Build history of the part. All positions in model axes, mm. A direction names the side the tool comes from. Round coordinates to 2 decimals unless told otherwise and drop trailing zeros. Loops run counter-clockwise (first coordinate to the right, second up) from the corner with the lowest first, then second, coordinate; pieces in that order, holes last. Notation, with made-up numbers: (59.5, 48) - (112.5, 48) arc R11 ccw to (112.5, 66) - close; hole circle Ø6 at (66.5, 42.25). An arc over 180 degrees is marked (long way). Put each result on its own line as item: value. Start each with the question number.
from build123d import *

# Parameters (mm, degrees)
SKETCH2_R                            = 3.35
F_40_SERIES_TS40_80LM_650037_1_DEPTH = 175


with BuildPart() as part:
    # Sketch2 → 40 series TS40-80LM-650037(1) (new body)
    with BuildSketch(Plane(origin=(0, 0, 0), x_dir=(-1, 0, 0), z_dir=(0, 1, 0))):
        with BuildLine():
            Line((0, -27.681), (-5.525738531, -27.681))
            Line((-5.525738531, -27.681), (-11.176, -33.331261469))
            Line((-11.176, -33.331261469), (-11.176, -36.6218))
            Line((-11.176, -36.6218), (-7.6835, -36.6218))
            Line((-7.6835, -36.6218), (-7.6835, -35.2248))
            Line((-7.6835, -35.2248), (-4.0488, -35.2248))
            Line((-4.0488, -35.2248), (-4.0488, -40))
            Line((-4.0488, -40), (-17, -40))
            ThreePointArc((-17, -40), (-19.121320344, -39.121320344), (-20, -37))
            Line((-20, -37), (-20, -24.0488))
            Line((-20, -24.0488), (-15.2248, -24.0488))
            Line((-15.2248, -24.0488), (-15.2248, -27.6835))
            Line((-15.2248, -27.6835), (-16.6218, -27.6835))
            Line((-16.6218, -27.6835), (-16.6218, -31.176))
            Line((-16.6218, -31.176), (-13.331261469, -31.176))
            Line((-13.331261469, -31.176), (-7.681, -25.525738531))
            Line((-7.681, -25.525738531), (-7.681, -20))
            Line((-7.681, -20), (-7.681, -14.474261469))
            Line((-7.681, -14.474261469), (-13.331261469, -8.824))
            Line((-13.331261469, -8.824), (-16.6218, -8.824))
            Line((-16.6218, -8.824), (-16.6218, -12.3165))
            Line((-16.6218, -12.3165), (-15.2248, -12.3165))
            Line((-15.2248, -12.3165), (-15.2248, -15.9512))
            Line((-15.2248, -15.9512), (-20, -15.9512))
            Line((-20, -15.9512), (-20, 15.9512))
            Line((-20, 15.9512), (-15.2248, 15.9512))
            Line((-15.2248, 15.9512), (-15.2248, 12.3165))
            Line((-15.2248, 12.3165), (-16.6218, 12.3165))
            Line((-16.6218, 12.3165), (-16.6218, 8.824))
            Line((-16.6218, 8.824), (-13.331261469, 8.824))
            Line((-13.331261469, 8.824), (-7.681, 14.474261469))
            Line((-7.681, 14.474261469), (-7.681, 25.525738531))
            Line((-7.681, 25.525738531), (-13.331261469, 31.176))
            Line((-13.331261469, 31.176), (-16.6218, 31.176))
            Line((-16.6218, 31.176), (-16.6218, 27.6835))
            Line((-16.6218, 27.6835), (-15.2248, 27.6835))
            Line((-15.2248, 27.6835), (-15.2248, 24.0488))
            Line((-15.2248, 24.0488), (-20, 24.0488))
            Line((-20, 24.0488), (-20, 37))
            ThreePointArc((-20, 37), (-19.121320344, 39.121320344), (-17, 40))
            Line((-17, 40), (-4.0488, 40))
            Line((-4.0488, 40), (-4.0488, 35.2248))
            Line((-4.0488, 35.2248), (-7.6835, 35.2248))
            Line((-7.6835, 35.2248), (-7.6835, 36.6218))
            Line((-7.6835, 36.6218), (-11.176, 36.6218))
            Line((-11.176, 36.6218), (-11.176, 33.331261469))
            Line((-11.176, 33.331261469), (-5.525738531, 27.681))
            Line((-5.525738531, 27.681), (0, 27.681))
            Line((0, 27.681), (5.525738531, 27.681))
            Line((5.525738531, 27.681), (11.176, 33.331261469))
            Line((11.176, 33.331261469), (11.176, 36.6218))
            Line((11.176, 36.6218), (7.6835, 36.6218))
            Line((7.6835, 36.6218), (7.6835, 35.2248))
            Line((7.6835, 35.2248), (4.0488, 35.2248))
            Line((4.0488, 35.2248), (4.0488, 40))
            Line((4.0488, 40), (17, 40))
            ThreePointArc((17, 40), (19.121320344, 39.121320344), (20, 37))
            Line((20, 37), (20, 24.0488))
            Line((20, 24.0488), (15.2248, 24.0488))
            Line((15.2248, 24.0488), (15.2248, 27.6835))
            Line((15.2248, 27.6835), (16.6218, 27.6835))
            Line((16.6218, 27.6835), (16.6218, 31.176))
            Line((16.6218, 31.176), (13.331261469, 31.176))
            Line((13.331261469, 31.176), (7.681, 25.525738531))
            Line((7.681, 25.525738531), (7.681, 20))
            Line((7.681, 20), (7.681, 14.474261469))
            Line((7.681, 14.474261469), (13.331261469, 8.824))
            Line((13.331261469, 8.824), (16.6218, 8.824))
            Line((16.6218, 8.824), (16.6218, 12.3165))
            Line((16.6218, 12.3165), (15.2248, 12.3165))
            Line((15.2248, 12.3165), (15.2248, 15.9512))
            Line((15.2248, 15.9512), (20, 15.9512))
            Line((20, 15.9512), (20, -15.9512))
            Line((20, -15.9512), (15.2248, -15.9512))
            Line((15.2248, -15.9512), (15.2248, -12.3165))
            Line((15.2248, -12.3165), (16.6218, -12.3165))
            Line((16.6218, -12.3165), (16.6218, -8.824))
            Line((16.6218, -8.824), (13.331261469, -8.824))
            Line((13.331261469, -8.824), (7.681, -14.474261469))
            Line((7.681, -14.474261469), (7.681, -20))
            Line((7.681, -20), (7.681, -25.525738531))
            Line((7.681, -25.525738531), (13.331261469, -31.176))
            Line((13.331261469, -31.176), (16.6218, -31.176))
            Line((16.6218, -31.176), (16.6218, -27.6835))
            Line((16.6218, -27.6835), (15.2248, -27.6835))
            Line((15.2248, -27.6835), (15.2248, -24.0488))
            Line((15.2248, -24.0488), (20, -24.0488))
            Line((20, -24.0488), (20, -37))
            ThreePointArc((20, -37), (19.121320344, -39.121320344), (17, -40))
            Line((17, -40), (4.0488, -40))
            Line((4.0488, -40), (4.0488, -35.2248))
            Line((4.0488, -35.2248), (7.6835, -35.2248))
            Line((7.6835, -35.2248), (7.6835, -36.6218))
            Line((7.6835, -36.6218), (11.176, -36.6218))
            Line((11.176, -36.6218), (11.176, -33.331261469))
            Line((11.176, -33.331261469), (5.525738531, -27.681))
            Line((5.525738531, -27.681), (0, -27.681))
        make_face()
        with Locations((0, -20)):
            Circle(SKETCH2_R, mode=Mode.SUBTRACT)
        with Locations((0, 20)):
            Circle(SKETCH2_R, mode=Mode.SUBTRACT)
        Polygon((-5.525738531, 12.319), (-17.844738531, 0), (-5.525738531, -12.319), (0, -12.319), (5.525738531, -12.319), (17.844738531, 0), (5.525738531, 12.319), (0, 12.319), align=None, mode=Mode.SUBTRACT)
        with BuildLine():
            Line((12.8372, 38.222), (12.8372, 32.8372))
            Line((12.8372, 32.8372), (18.222, 32.8372))
            Line((18.222, 32.8372), (18.222, 35.428))
            ThreePointArc((18.222, 35.428), (17.403656347, 37.403656347), (15.428, 38.222))
            Line((15.428, 38.222), (12.8372, 38.222))
        make_face(mode=Mode.SUBTRACT)
        with BuildLine():
            Line((12.8372, -32.8372), (18.222, -32.8372))
            Line((18.222, -32.8372), (18.222, -35.428))
            ThreePointArc((18.222, -35.428), (17.403656347, -37.403656347), (15.428, -38.222))
            Line((15.428, -38.222), (12.8372, -38.222))
            Line((12.8372, -38.222), (12.8372, -32.8372))
        make_face(mode=Mode.SUBTRACT)
        with BuildLine():
            Line((-12.8372, -38.222), (-12.8372, -32.8372))
            Line((-12.8372, -32.8372), (-18.222, -32.8372))
            Line((-18.222, -32.8372), (-18.222, -35.428))
            ThreePointArc((-18.222, -35.428), (-17.403656347, -37.403656347), (-15.428, -38.222))
            Line((-15.428, -38.222), (-12.8372, -38.222))
        make_face(mode=Mode.SUBTRACT)
        with BuildLine():
            Line((-18.222, 35.428), (-18.222, 32.8372))
            Line((-18.222, 32.8372), (-12.8372, 32.8372))
            Line((-12.8372, 32.8372), (-12.8372, 38.222))
            Line((-12.8372, 38.222), (-15.428, 38.222))
            ThreePointArc((-15.428, 38.222), (-17.403656347, 37.403656347), (-18.222, 35.428))
        make_face(mode=Mode.SUBTRACT)
    extrude(amount=F_40_SERIES_TS40_80LM_650037_1_DEPTH)


solid = part.part
Item 1: Slice it at B-B (x = 0). Give the cut face in (y, z), plus the area to 3 significant figures.
Item 2: Drop flat-ended pins along their axis: pin 1 Ø1.5 at (x, y) = (2.5, 90.5) entering from -Z; pin 2 Ø5.5 at (y, z) = (121, -19.5) entering from -X. Give the stop position or say it passes through.
Item 3: Drill centre lines: probe 1 along Z at (x, y) = (0, 104.5); probe 2 along X at (y, z) = (32.5, 30); probe 3 along Z at (x, y) = (-7.5, 76). Where is each one in solid material? Low to high. Write a range as [from, to].
Item 4: Two-plate mould, pull along Z, no slides. Class faces 3 (the flat face through (-4.049, 86, -38)), 4 (the cylindrical face through (-19.1, 86.28, 39.14)), 5 (the flat face through (15.225, 86, -26)), 6 (the flat face through (15, 86, -32.837)): pulls with the +Z half, pulls with the -Z half, needs draft (parallel to the pull), parting line crosses it, or undercut.
Item 5: Slice it at A-A (z = 20). Give the cut face in (x, y), plus the area to 3 significant figures.
Item 6: Slice it at C-C (y = 135.5). Give the number of separate pieces and of enclosed holes in the cut face, plus the area to 3 significant figures.
Item 7: Which spindle directions (+Z, -Z, +X, -X, +Y, -Y) get a long thin tool onto all of the face, cutting with end or side? Do faces 1 (the flat face through (18, 86, 15.951)), 2 (the flat face through (-15.225, 86, -26)). Say none if no direction does.
Computed values:
1. outline: (0, -27.68) - (175, -27.68) - (175, -23.35) - (0, -23.35) - close; (0, -16.65) - (175, -16.65) - (175, -12.32) - (0, -12.32) - close; (0, 12.32) - (175, 12.32) - (175, 16.65) - (0, 16.65) - close; (0, 23.35) - (175, 23.35) - (175, 27.68) - (0, 27.68) - close
1. area: 3,030 mm^2
2. pin 1: stops at z = -27.68
2. pin 2: stops at x = -7.68
3. probe 1: z = [-27.68, -23.35], [-16.65, -12.32], [12.32, 16.65], [23.35, 27.68]
3. probe 2: x = [-20, -16.62], [-12.16, -7.84], [7.84, 12.16], [16.62, 20]
3. probe 3: z = [-40, -35.22], [-29.66, -10.34], [10.34, 29.66], [35.22, 40]
4. face 3: needs draft
4. face 4: pulls with the +Z half
4. face 5: undercut
4. face 6: undercut
5. outline: (-7.68, 0) - (-3.35, 0) - (-3.35, 175) - (-7.68, 175) - close; (3.35, 0) - (7.68, 0) - (7.68, 175) - (3.35, 175) - close
5. area: 1,520 mm^2
6. separate pieces: 1
6. enclosed holes: 7
6. area: 1,330 mm^2
7. face 1: +X, +Y, -Y
7. face 2: +Y, -Y
